Here's how the part is built. I have some questions about the finished solid (model axes, mm). A direction names the side the tool comes from. Round coordinates to 2 decimals unless told otherwise and drop trailing zeros. Write each loop counter-clockwise with the first axis right and the second up, starting at its lowest first coordinate (ties: lowest second). Pieces come first, ordered by that corner, then holes. Notation, with made-up numbers: (79.5, -7) - (89.5, -7) arc R18 cw to (89.5, 20) - close; hole circle Ø7 at (21, 80). An arc over 180 degrees is marked (long way). Write item = value, one per line. Start each with the question number.
Item 1: Which directions (+Z, -Z, +X, -X, +Y, -Y) give clear straight access to the entire face, cutting with the end or side of a thin tool? Please do faces 1 (the face through (-65.361, 19.243, 4.412)), 2 (the face through (-62, 8, -1)), 3 (the face through (-48.25, 17.2, -0.4)).
Item 2: For P1, Ø4, axis at x = -16, y = -8, coming from the +Z side; P2, Ø1.6, axis at x = 39.5, z = -0.5, coming from the +Y side, each with a flat end and sliding along its axis, tell me the tip position at first contact or that it passes through.
Item 3: If we section it at C-C (x = -8): Please give me the cut outline in (y, z), and give its area (3 significant figures).
Item 4: If we section it at B-B (x = -62): Please give me the cut outline in (y, z).
Item 5: If I drill on line 1 along X through (y, z) = (15.5, -1.5); line 2 along Z through (x, y) = (-58, 17.5); line 3 along Z through (x, y) = (-15.5, -3.5), over which ranges is the centre line in solid material (lowest first)? Write a range as [from, to].
Item 6: Thinking about a two-plate mould opening in Z: for faces 4 (the face through (82, 9, -1)), 5 (the face through (64.889, 19.243, 4.412)), 6 (the face through (-65.36, 20.82, 5.66)), which applies, pulls with the +Z half, pulls with the -Z half, needs draft (parallel to the pull), parting line crosses it, or undercut?
Item 7: If we section it at D-D (y = -7.5): Please give me the cut outline in (x, z).
Item 8: If we section it at A-A (y = 2.5): Please give me the cut outline in (x, z), and give its area (3 significant figures).
```python
from build123d import *

# Parameters (mm, degrees)
BASIS_BLECH1_DEPTH       = 2
BLECHKANTENRAND1_START   = -82
BLECHKANTENRAND1_DEPTH   = 33.75
BLECHKANTENRAND1_START_2 = 48.25
BLECHKANTENRAND1_2_DEPTH = 33.75
BLECHKANTENRAND1_START_3 = -15.75
BLECHKANTENRAND1_3_DEPTH = 31.5


# Read off the part's stored shape, not the designer's step: Blechkantenrand1
# Sheet-metal steps are written as plain solids
with BuildPart() as part:
    # Skizze1 → Basis-Blech1 (new body)
    with BuildSketch(Plane.XY):
        Polygon((-82, 12.5), (-82, 17.5), (-48.25, 17.5), (-48.25, 12.5), (-15.75, 12.5), (-15.75, 17.5), (15.75, 17.5), (15.75, 12.5), (48.25, 12.5), (48.25, 17.5), (82, 17.5), (82, 12.5), (82, -12.5), (-82, -12.5), align=None)
        with BuildLine():
            Line((-58.5, 4.5), (-58.5, -5.5))
            ThreePointArc((-58.5, -5.5), (-62, -9), (-65.5, -5.5))
            Line((-65.5, -5.5), (-65.5, 4.5))
            ThreePointArc((-65.5, 4.5), (-62, 8), (-58.5, 4.5))
        make_face(mode=Mode.SUBTRACT)
        with BuildLine():
            Line((65.5, 4.5), (65.5, -5.5))
            ThreePointArc((65.5, -5.5), (62, -9), (58.5, -5.5))
            Line((58.5, -5.5), (58.5, 4.5))
            ThreePointArc((58.5, 4.5), (62, 8), (65.5, 4.5))
        make_face(mode=Mode.SUBTRACT)
    extrude(amount=-BASIS_BLECH1_DEPTH)

    # Blechkantenrand1 outline → Blechkantenrand1 (add)
    with BuildSketch(Plane.YZ.offset(BLECHKANTENRAND1_START)):
        with BuildLine():
            Line((12.95, 2.55), (14.95, 2.55))
            ThreePointArc((14.95, 2.55), (19.303122292, 4.353122292), (17.5, 0))
            Line((17.5, 0), (17.5, -2))
            ThreePointArc((17.5, -2), (20.717335854, 5.767335854), (12.95, 2.55))
        make_face()
    extrude(amount=BLECHKANTENRAND1_DEPTH)

    # Blechkantenrand1 2 outline → Blechkantenrand1 2 (add)
    with BuildSketch(Plane.YZ.offset(BLECHKANTENRAND1_START_2)):
        with BuildLine():
            Line((12.95, 2.55), (14.95, 2.55))
            ThreePointArc((14.95, 2.55), (19.303122292, 4.353122292), (17.5, 0))
            Line((17.5, 0), (17.5, -2))
            ThreePointArc((17.5, -2), (20.717335854, 5.767335854), (12.95, 2.55))
        make_face()
    extrude(amount=BLECHKANTENRAND1_2_DEPTH)

    # Blechkantenrand1 3 outline → Blechkantenrand1 3 (add)
    with BuildSketch(Plane.YZ.offset(BLECHKANTENRAND1_START_3)):
        with BuildLine():
            Line((12.95, 2.55), (14.95, 2.55))
            ThreePointArc((14.95, 2.55), (19.303122292, 4.353122292), (17.5, 0))
            Line((17.5, 0), (17.5, -2))
            ThreePointArc((17.5, -2), (20.717335854, 5.767335854), (12.95, 2.55))
        make_face()
    extrude(amount=BLECHKANTENRAND1_3_DEPTH)


solid = part.part
```
Reply:
q1.face_1 = +X, -X
q1.face_2 = +Z, -Z
q1.face_3 = +Z, -Z, +Y
q2.P1 = 0
q2.P2 = 12.5
q3.outline = (-12.5, -2) - (17.5, -2) arc R4.55 ccw (long way) to (12.95, 2.55) - (14.95, 2.55) arc R2.55 cw (long way) to (17.5, 0) - (-12.5, 0) - close
q3.area = 93.5 mm2
q4.outline = (-12.5, -2) - (-9, -2) - (-9, 0) - (-12.5, 0) - close; (8, -2) - (17.5, -2) arc R4.55 ccw (long way) to (12.95, 2.55) - (14.95, 2.55) arc R2.55 cw (long way) to (17.5, 0) - (8, 0) - close
q5.line_1 = [-82, -48.25], [-15.75, 15.75], [48.25, 82]
q5.line_2 = [-2, 0], [5.1, 7.1]
q5.line_3 = [-2, 0]
q6.face_4 = needs draft
q6.face_5 = undercut
q6.face_6 = parting line crosses it
q7.outline = (-82, -2) - (-64.87, -2) - (-64.87, 0) - (-82, 0) - close; (-59.13, -2) - (59.13, -2) - (59.13, 0) - (-59.13, 0) - close; (64.87, -2) - (82, -2) - (82, 0) - (64.87, 0) - close
q8.outline = (-82, -2) - (-65.5, -2) - (-65.5, 0) - (-82, 0) - close; (-58.5, -2) - (58.5, -2) - (58.5, 0) - (-58.5, 0) - close; (65.5, -2) - (82, -2) - (82, 0) - (65.5, 0) - close
q8.area = 300 mm2
